Verification items for the finished model (mm, model axes). A direction names the side the tool comes from. Give positions to 0.01 mm unless a question says otherwise; leave off trailing zeros. Loops run counter-clockwise (first coordinate to the right, second up) from the corner with the lowest first, then second, coordinate; pieces in that order, holes last. Notation, with made-up numbers: M -7,-27.5 L 12,-27.5 A27 ccw 12,-7.5 Z; hole C 26.5,-38.75 d2. An arc over 180 degrees is marked long. Use CSV: the item, a comma, the result in double quotes.
from build123d import *

# Parameters (mm, degrees)
SKETCH1_W           = 30.2
SKETCH1_H           = 32.2
BOSS_EXTRUDE1_DEPTH = 10
FILLET1_R           = 1.5
SKETCH3_R           = 3.15
CUT_EXTRUDE1_DEPTH  = 71.165803637
SKETCH6_W           = 53.8
SKETCH6_H           = 56.6
CUT_EXTRUDE4_DEPTH  = 59.998389809
SKETCH4_R           = 7
CUT_EXTRUDE2_DEPTH  = 32.3
FILLET2_R           = 3
FILLET3_R           = 4
CHAMFER1_SIZE       = 0.5
SKETCH5_R           = 2.5
CUT_EXTRUDE3_DEPTH  = 71.165803637


with BuildPart() as part:
    # Sketch1 → Boss-Extrude1 (new, symmetric)
    with BuildSketch(Plane.XY):
        Polygon((-50, -14.2), (-29.5, -14.2), (-23.1, -20.6), (-23.1, -24.1), (23.1, -24.1), (23.1, -20.6), (29.5, -14.2), (50, -14.2), (50, 24.1), (-50, 24.1), align=None)
        Rectangle(SKETCH1_W, SKETCH1_H, mode=Mode.SUBTRACT)
    extrude(amount=BOSS_EXTRUDE1_DEPTH, both=True)

    # Fillet1
    fillet1_edges = [part.edges().sort_by_distance(p)[0] for p in [
        (15.1, -16.1, 0),
        (15.1, 16.1, 0),
        (-15.1, 16.1, 0),
        (-15.1, -16.1, 0),
    ]]
    fillet(fillet1_edges, radius=FILLET1_R)

    # Sketch3 → Cut-Extrude1 (cut, through all)
    with BuildSketch(Plane(origin=(0, 24.1, 0), x_dir=(1, 0, 0), z_dir=(0, 1, 0))):
        with Locations(Location((-40, 0, 0), (0, 0, 270))):
            Circle(SKETCH3_R)
        with Locations(Location((40, 0, 0), (0, 0, 270))):
            Circle(SKETCH3_R)
    extrude(amount=-CUT_EXTRUDE1_DEPTH, mode=Mode.SUBTRACT)

    # Sketch6 → Cut-Extrude4 (cut, through all)
    with BuildSketch(Plane.XY.offset(10)):
        with Locations((-50, 24.1)):
            Rectangle(SKETCH6_W, SKETCH6_H)
        with Locations((50, 24.1)):
            Rectangle(SKETCH6_W, SKETCH6_H)
    extrude(amount=-CUT_EXTRUDE4_DEPTH, mode=Mode.SUBTRACT)

    # Sketch4 → Cut-Extrude2 (cut)
    with BuildSketch(Plane(origin=(0, 24.1, 0), x_dir=(1, 0, 0), z_dir=(0, 1, 0))):
        with Locations(Location((-40, 0, 0), (0, 0, 270))):
            Circle(SKETCH4_R)
        with Locations(Location((40, 0, 0), (0, 0, 270))):
            Circle(SKETCH4_R)
    extrude(amount=-CUT_EXTRUDE2_DEPTH, mode=Mode.SUBTRACT)

    # Fillet2
    fillet2_edges = [part.edges().sort_by_distance(p)[0] for p in [
        (23.1, -24.1, 0),
        (-23.1, -24.1, 0),
        (23.1, 24.1, 0),
        (-23.1, 24.1, 0),
    ]]
    fillet(fillet2_edges, radius=FILLET2_R)

    # Fillet3
    fillet3_edges = [part.edges().sort_by_distance(p)[0] for p in [
        (23.1, -4.2, 0),
        (-23.1, -4.2, 0),
    ]]
    fillet(fillet3_edges, radius=FILLET3_R)

    # Chamfer1
    chamfer1_edges = [part.edges().sort_by_distance(p)[0] for p in [
        (50, -4.2, 0),
        (50, -9.2, -10),
        (39.75, -14.2, -10),
        (26.3, -17.4, -10),
        (-23.1, -20.85, -10),
        (-26.3, -17.4, 10),
        (-26.3, -17.4, -10),
        (-39.75, -14.2, -10),
        (0, 24.1, -10),
        (0, 24.1, 10),
        (23.1, 10.45, -10),
        (23.1, -20.85, -10),
        (0, -24.1, -10),
        (-22.221320344, -23.221320344, -10),
        (22.221320344, -23.221320344, -10),
        (-22.221320344, 23.221320344, -10),
        (22.221320344, 23.221320344, -10),
        (23.1, 10.45, 10),
        (0, -24.1, 10),
        (23.1, -20.85, 10),
        (-22.221320344, -23.221320344, 10),
        (22.221320344, -23.221320344, 10),
        (-22.221320344, 23.221320344, 10),
        (22.221320344, 23.221320344, 10),
        (38.55, -4.2, -10),
        (38.55, -4.2, 10),
        (-23.1, 10.45, 10),
        (-23.1, 10.45, -10),
        (24.271572875, -3.028427125, 10),
        (-23.1, -20.85, 10),
        (24.271572875, -3.028427125, -10),
        (-24.271572875, -3.028427125, 10),
        (-24.271572875, -3.028427125, -10),
        (50, -14.2, 0),
        (-50, -14.2, 0),
        (26.3, -17.4, 10),
        (39.75, -14.2, 10),
        (50, -9.2, 10),
        (-15.1, 0, -10),
        (-15.1, 0, 10),
        (0, -16.1, -10),
        (0, -16.1, 10),
        (15.1, 0, -10),
        (15.1, 0, 10),
        (0, 16.1, -10),
        (0, 16.1, 10),
        (-14.660660172, -15.660660172, -10),
        (-14.660660172, -15.660660172, 10),
        (14.660660172, -15.660660172, -10),
        (14.660660172, -15.660660172, 10),
        (14.660660172, 15.660660172, -10),
        (14.660660172, 15.660660172, 10),
        (-14.660660172, 15.660660172, -10),
        (-14.660660172, 15.660660172, 10),
        (-50, -9.2, -10),
        (-50, -9.2, 10),
        (-38.55, -4.2, 10),
        (-39.75, -14.2, 10),
        (-50, -4.2, 0),
        (-38.55, -4.2, -10),
    ]]
    chamfer(chamfer1_edges, length=CHAMFER1_SIZE)

    # Sketch5 → Cut-Extrude3 (cut, through all)
    with BuildSketch(Plane(origin=(0, 24.1, 0), x_dir=(1, 0, 0), z_dir=(0, 1, 0))):
        with Locations(Location((0, 0, 0), (0, 0, 270))):
            Circle(SKETCH5_R)
    extrude(amount=-CUT_EXTRUDE3_DEPTH, mode=Mode.SUBTRACT)


solid = part.part
(1) Section check D-D on y = -7. Record the cut outline in (x, z).
Calculated:
outline,"M -50,-9.5 L -49.5,-10 L -15.6,-10 L -15.1,-9.5 L -15.1,9.5 L -15.6,10 L -49.5,10 L -50,9.5 Z; M 15.1,-9.5 L 15.6,-10 L 49.5,-10 L 50,-9.5 L 50,9.5 L 49.5,10 L 15.6,10 L 15.1,9.5 Z; hole C -40,0 d14; hole C 40,0 d14"
(2) Mould release check, pull along Y, two halves, no side actions. Record for faces 1 (the flat face through (33, -4.2, 2)), 2 (the flat face through (-23.1, 10, 0)), 3 (the conical face through (14.75, 15.77, -9.64)), 4 (the conical face through (-21.989, -22.948, 9.858)): released by +Y, released by -Y, zero draft, split by the parting line, or undercut.
Calculated:
face 1,"released by +Y"
face 2,"zero draft"
face 3,"undercut"
face 4,"released by -Y"
(3) Scan lines: L1, parallel to X at y = -11.8, z = 0; L2, parallel to X at y = 9, z = 0.75; L3, parallel to Y at x = 12.5, z = 1.25. Record each from-to range of solid material in increasing order. Write a range as from..to.
Calculated:
L1,"x = -50..-43.15, -36.85..-15.1, 15.1..36.85, 43.15..50"
L2,"x = -23.1..-15.1, 15.1..23.1"
L3,"y = -24.1..-16.1, 16.1..24.1"
(4) Section check C-C on y = 10.5. Record the cut outline in (x, z), plus the area to 3 significant figures.
Calculated:
outline,"M -23.1,-9.5 L -22.6,-10 L -15.6,-10 L -15.1,-9.5 L -15.1,9.5 L -15.6,10 L -22.6,10 L -23.1,9.5 Z; M 15.1,-9.5 L 15.6,-10 L 22.6,-10 L 23.1,-9.5 L 23.1,9.5 L 22.6,10 L 15.6,10 L 15.1,9.5 Z"
area,"319 mm²"
(5) Depth check by flat-ended pin: pin 1 Ø3 at (x, z) = (-23.5, -6.5) entering from +Y; pin 2 Ø5.5 at (x, z) = (43, -3.5) entering from -Y; pin 3 Ø5.5 at (y, z) = (5.5, -1) entering from +X; pin 4 Ø10 at (x, y) = (4, 9.5) entering from +Z. Enter the tip coordinate at first touch or a pass-through.
Calculated:
pin 1,"stops at y = 23.42"
pin 2,"stops at y = -14.2"
pin 3,"stops at x = 23.1"
pin 4,"passes through"
(6) Section check B-B on x = -3.5. Record the cut outline in (y, z).
Calculated:
outline,"M -24.1,-9.5 L -23.6,-10 L -16.6,-10 L -16.1,-9.5 L -16.1,9.5 L -16.6,10 L -23.6,10 L -24.1,9.5 Z; M 16.1,-9.5 L 16.6,-10 L 23.6,-10 L 24.1,-9.5 L 24.1,9.5 L 23.6,10 L 16.6,10 L 16.1,9.5 Z"
(7) Tool access check on faces 5 (the flat face through (-41.5, -8.2, 3)), 6 (the conical face through (14.744, 15.769, 9.635)), 7 (the flat face through (-37, -14.2, 2)), 8 (the flat face through (-33, -4.2, 4)). Record the directions out of +Z, -Z, +X, -X, +Y, -Y that give a thin tool (end or side, any length) a straight path to the whole face; none if there is none.
Calculated:
face 5,"+Y"
face 6,"+Z"
face 7,"+Z, -Z, -X, -Y"
face 8,"+Z, -Z, -X, +Y"
(8) Section check A-A on y = -12. Record the cut outline in (x, z).
Calculated:
outline,"M -50,-9.5 L -49.5,-10 L -15.6,-10 L -15.1,-9.5 L -15.1,9.5 L -15.6,10 L -49.5,10 L -50,9.5 Z; M 15.1,-9.5 L 15.6,-10 L 49.5,-10 L 50,-9.5 L 50,9.5 L 49.5,10 L 15.6,10 L 15.1,9.5 Z; hole C -40,0 d6.3; hole C 40,0 d6.3"
